from build123d import *

# Parameters (mm, degrees)
SKETCH_1_R               = 8.8
EXTRUDE_1_DEPTH          = 6
SKETCH_6_W               = 0.7
SKETCH_6_H               = 6
REVOLVE_1_ANGLE          = 5
PATTERN_CIRCULAR_5_COUNT = 2
SKETCH_7_R               = 8.7
EXTRUDE_10_DEPTH         = 46.6
SKETCH_8_R               = 4.5
EXTRUDE_11_DEPTH         = 1.4
SKETCH_9_R               = 1.5
EXTRUDE_12_DEPTH         = 12
F_2_0MM_1_D              = 2
F_2_0MM_1_DEPTH          = 5
F_2_0MM_1_TIP            = 0.600860619
F_2_0MM_2_D              = 2
F_2_0MM_2_DEPTH          = 5
F_2_0MM_2_TIP            = 0.600860619


with BuildPart() as part:
    # 草图1 → 凸台-拉伸1 (new body)
    with BuildSketch(Plane(origin=(0, 0, 0), x_dir=(1, 0, 0), z_dir=(0, 1, 0))):
        with Locations(Location((0, 0, 0), (0, 0, 270))):
            Circle(SKETCH_1_R)
    extrude(amount=EXTRUDE_1_DEPTH)

    # 草图6 → 旋转1 (revolve, symmetric)
    with BuildSketch(Plane.XY) as revolve_1_sk:
        with Locations((-9.15, 3)):
            Rectangle(SKETCH_6_W, SKETCH_6_H)
    revolve_1 = revolve(axis=Axis((0, 1.183639986, 0), (0, -1, 0)), revolution_arc=REVOLVE_1_ANGLE / 2)
    revolve_1 = revolve_1 + revolve(revolve_1_sk.sketch, axis=Axis((0, 1.183639986, 0), (0, 1, 0)), revolution_arc=REVOLVE_1_ANGLE / 2)

    # 阵列(圆周)5: 旋转1 ×2 about axis
    pattern_circular_5_axis = Axis((0, 0, 0), (0, 1, 0))
    for i in range(1, PATTERN_CIRCULAR_5_COUNT):
        add(revolve_1.rotate(pattern_circular_5_axis, i * 360 / PATTERN_CIRCULAR_5_COUNT))

    # 草图7 → 凸台-拉伸10 (add)
    with BuildSketch(Plane(origin=(0, 6, 0), x_dir=(1, 0, 0), z_dir=(0, 1, 0))):
        with Locations(Location((0, 0, 0), (0, 0, 270))):
            Circle(SKETCH_7_R)
    extrude(amount=EXTRUDE_10_DEPTH)

    # 草图8 → 凸台-拉伸11 (add)
    with BuildSketch(Plane(origin=(0, 52.6, 0), x_dir=(1, 0, 0), z_dir=(0, 1, 0))):
        with Locations(Location((0, 0, 0), (0, 0, 270))):
            Circle(SKETCH_8_R)
    extrude(amount=EXTRUDE_11_DEPTH)

    # 草图9 → 凸台-拉伸12 (add)
    with BuildSketch(Plane(origin=(0, 54, 0), x_dir=(1, 0, 0), z_dir=(0, 1, 0))):
        with Locations(Location((0, 0, 0), (0, 0, 270))):
            Circle(SKETCH_9_R)
    extrude(amount=EXTRUDE_12_DEPTH)

    # Ø2.0mm 暗销孔1
    with Locations(Plane(origin=(-6.72, 0, 0), x_dir=(0, 0, -1), z_dir=(0, -1, 0))):
        with Locations((0, 0)):
            Hole(F_2_0MM_1_D / 2, depth=F_2_0MM_1_DEPTH)
            with Locations((0, 0, -(F_2_0MM_1_DEPTH + F_2_0MM_1_TIP / 2))):  # 118° drill point
                Cone(0, F_2_0MM_1_D / 2, F_2_0MM_1_TIP, mode=Mode.SUBTRACT)

    # Ø2.0mm 暗销孔2
    with Locations(Plane(origin=(6.72, 0, 0), x_dir=(0, 0, -1), z_dir=(0, -1, 0))):
        with Locations((0, 0)):
            Hole(F_2_0MM_2_D / 2, depth=F_2_0MM_2_DEPTH)
            with Locations((0, 0, -(F_2_0MM_2_DEPTH + F_2_0MM_2_TIP / 2))):  # 118° drill point
                Cone(0, F_2_0MM_2_D / 2, F_2_0MM_2_TIP, mode=Mode.SUBTRACT)


solid = part.part
Part model, mm, in its own coordinate system. A direction names the side the tool comes from. Coordinates: 2 decimals unless noted, no trailing zeros. Write each loop counter-clockwise with the first axis right and the second up, starting at its lowest first coordinate (ties: lowest second). Pieces come first, ordered by that corner, then holes. Notation, with made-up numbers: (40, -26) - (71, -26) arc R31 cw to (71, 1) - close; hole circle Ø4 at (61.5, 70.25). An arc over 180 degrees is marked (long way). Put each result on its own line as item: value.
1. Band-saw the part on C-C (y = 57.5). Write the cut outline in (x, z), then the cut area to 3 significant figures.
Final values:
outline: circle Ø3 at (0, 0)
area: 7.07 mm²
2. 3-axis set-ups, long thin cutter, end or side, ignore diameter. For faces 5 (the flat face through (-2, 54, 0)), 6 (the cylindrical face through (-5.73, 2.54, -0.13)), 7 (the flat face through (0, 0, 0)): which of +Z, -Z, +X, -X, +Y, -Y reach the whole face in a straight line?
Final values:
face 5: +Y
face 6: -Y
face 7: +Z, -Z, +X, -X, -Y
3. Flat gauge pins, fed straight in: pin 1 Ø8 at (y, z) = (17.5, -3.5) entering from +X; pin 2 Ø2 at (x, z) = (7, -5) entering from +Y; pin 3 Ø1.8 at (x, z) = (6.72, 0) entering from -Y. Where does each tip first touch, or does it go through?
Final values:
pin 1: stops at x = 8.7
pin 2: stops at y = 52.6
pin 3: stops at y = 5.06
4. Band-saw the part on B-B (z = -6.75). Write the cut outline in (x, y), then the cut area to 3 significant figures.
Final values:
outline: (-5.65, 0) - (5.65, 0) - (5.65, 6) - (5.49, 6) - (5.49, 52.6) - (-5.49, 52.6) - (-5.49, 6) - (-5.65, 6) - close
area: 579 mm²
5. Band-saw the part on D-D (z = 3.5). Write the cut outline in (x, y).
Final values:
outline: (-8.07, 0) - (8.07, 0) - (8.07, 6) - (7.96, 6) - (7.96, 52.6) - (2.83, 52.6) - (2.83, 54) - (-2.83, 54) - (-2.83, 52.6) - (-7.96, 52.6) - (-7.96, 6) - (-8.07, 6) - close
6. Two-plate mould, pull along Z, no slides. Class faces 1 (the cylindrical face through (-5.3, 29, -6.9)), 2 (the conical face through (-6.89, 5.497, 0.038)), 3 (the cylindrical face through (-0.188, 2.958, 8.798)), 4 (the flat face through (9, 6, 0)): +Z half, -Z half, draft (parallel to the pull), parting line (faces both ways), or undercut.
Final values:
face 1: parting line
face 2: undercut
face 3: +Z half
face 4: draft
7. Band-saw the part on A-A (x = 0). Write the cut outline in (y, z), then the cut area to 3 significant figures.
Final values:
outline: (0, -8.8) - (6, -8.8) - (6, -8.7) - (52.6, -8.7) - (52.6, -4.5) - (54, -4.5) - (54, -1.5) - (66, -1.5) - (66, 1.5) - (54, 1.5) - (54, 4.5) - (52.6, 4.5) - (52.6, 8.7) - (6, 8.7) - (6, 8.8) - (0, 8.8) - close
area: 965 mm²
8. Probe line 1 along X through (y, z) = (4.05, 0); line 2 along Y through (x, z) = (-0.5, 3); line 3 along Y through (x, z) = (3.75, -5.5). List the from-to ranges inside material, lowest first. Write a range as [from, to].
Final values:
line 1: x = [-9.5, -7.72], [-5.72, 5.72], [7.72, 9.5]
line 2: y = [0, 54]
line 3: y = [0, 52.6]
